Source: three-view drawing plus pictorial views. Frame: mm from the lowest corner of the part. A direction names the side the tool comes from. Give positions to 0.01 mm unless a question says otherwise; leave off trailing zeros. Order: outer loops, then holes, each group sorted by start corner. A loop starts at its lowest first (then second) coordinate and runs counter-clockwise, first axis right, second up. Notation, with made-up numbers: (75, -34.75) - (81, -34.75) arc R34 cw to (81, -4.75) - close; hole circle Ø5 at (8.25, 78). An arc over 180 degrees is marked (long way). Answer in a Markdown table with one row per item. Add a question column.
1. Access query for the marked faces 1 and 2. Directions: +Z, -Z, +X, -X, +Y, -Y. A direction counts if a zero-diameter tool reaches every point of the face in a straight line with its end or side. Return the directions, or none.
2. Section query C-C on z = 29. Return loops of the section in (x, y), and give its area (3 significant figures).
3. Section query A-A on y = 11. Return loops of the section in (x, z).
4. Ray query, line 1 (Z direction, x = 29, y = 1); line 2 (X direction, y = 1, z = 25.5). Return the intervals inside material, ascending. Write a range as [from, to].
5. Section query B-B on x = 25. Return loops of the section in (y, z), and give its area (3 significant figures).
6. Contact query for a flat-ended pin moving along its axis: pin 1 (6 mm diameter, centred on x = 19.5, y = 8.5, fed in from +Z). Output: stop coordinate, or through.
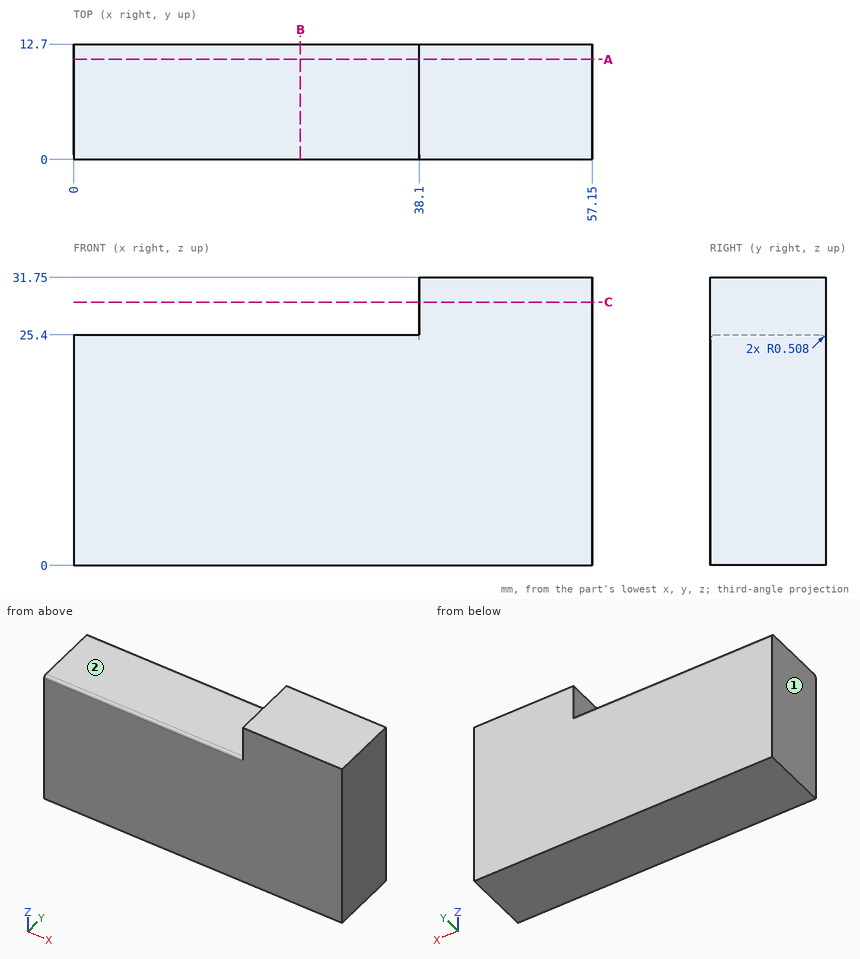
Answer:
| question | item | result |
|---|---|---|
| 1 | face 1 | +Z, -Z, -X, +Y, -Y |
| 1 | face 2 | +Z, -X, +Y, -Y |
| 2 | outline | (38.1, 0) - (57.15, 0) - (57.15, 12.7) - (38.1, 12.7) - close |
| 2 | area | 242 mm² |
| 3 | outline | (0, 0) - (57.15, 0) - (57.15, 31.75) - (38.1, 31.75) - (38.1, 25.4) - (0, 25.4) - close |
| 4 | line 1 | z = [0, 25.4] |
| 4 | line 2 | x = [38.1, 57.15] |
| 5 | outline | (0, 0) - (12.7, 0) - (12.7, 24.89) arc R0.51 ccw to (12.19, 25.4) - (0.51, 25.4) arc R0.51 ccw to (0, 24.89) - close |
| 5 | area | 322 mm² |
| 6 | pin 1 | stops at z = 25.4 |
